Work out the finished part from the listing and answer in its coordinate system (mm). Coordinates: 2 decimals unless noted, no trailing zeros. Write each loop counter-clockwise with the first axis right and the second up, starting at its lowest first coordinate (ties: lowest second). Pieces come first, ordered by that corner, then holes. Notation, with made-up numbers: (-16.75, 12) - (35.25, 12) arc R14 cw to (35.25, 16) - close; hole circle Ø5 at (62, 82). An arc over 180 degrees is marked (long way). Use a Markdown table: item, result. Add a question column.
(1) For a pull along Y with two mould halves and no side action, classify faces 1 (the face through (100.15, 47.07, 2.03)), 2 (the face through (66, 0, 2)) as released by +Y, released by -Y, zero draft, split by the parting line, or undercut.
(2) The part is cut by section B-B, the plane y = 35. Give the vertices of the cut face in (x, z).
(3) The part is cut by section D-D, the plane x = 101.75. Give the vertices of the cut face in (y, z), then the cut area to 3 significant figures.
(4) Find the intervals of material crossed by line 1 (X direction, y = 34, z = 3.25); line 2 (Y direction, x = 53.75, z = 1.45); line 3 (Y direction, x = 101.75, z = 2.45), in increasing order. Write a range as from..to.
(5) The part is cut by section A-A, the plane x = 125. Give the vertices of the cut face in (y, z).
(6) Given pin 1 Ø5 at (x, y) = (89.75, 47) entering from +Z, flat-ended and moving along its own axis, determine where the tip first touches the part or whether it passes through.
(7) The part is cut by section C-C, the plane x = 77.75. Give the vertices of the cut face in (y, z), then the cut area to 3 significant figures.
Autodesk Inventor part; units mm, degrees
ref_plane "YZ Plane" through (0, 0, 0) normal (1, 0, 0) x (0, 1, 0)
ref_plane "XZ Plane" through (0, 0, 0) normal (0, 1, 0) x (-1, 0, 0)
ref_plane "XY Plane" through (0, 0, 0) normal (0, 0, 1) x (1, 0, 0)
sketch "스케치1" plane through (0, 0, 0) normal (0, 0, 1) x (1, 0, 0)
  line L0 (0, 0) -> (0, 58)
  line L1 (0, 58) -> (129.5, 58)
  line L2 (129.5, 58) -> (129.5, 0)
  line L3 (129.5, 0) -> (0, 0)
  dimension "d0" = 58
  dimension "d1" = 129.5
extrude "돌출1" add sketch "스케치1" along normal blind 4
sketch "스케치2" plane through (0, 0, 4) normal (0, 0, 1) x (1, 0, 0)
  line L0 (62.75, 50) -> (62.75, 8)
  line L1 (32.75, 50) -> (57.25, 50)
  line L2 (62.75, 50) -> (69.25, 50)
  line L3 (81.25, 8) -> (81.25, 50)
  line L4 (74.75, 50) -> (81.25, 50)
  line L5 (74.75, 50) -> (74.75, 8)
  line L6 (74.75, 8) -> (81.25, 8)
  circle A0 centre (77.75, 47) radius 1.6
  circle A1 centre (77.75, 11) radius 1.6
  line L7 (93.25, 8) -> (93.25, 50)
  line L8 (86.75, 50) -> (93.25, 50)
  line L9 (86.75, 50) -> (86.75, 8)
  line L10 (86.75, 8) -> (93.25, 8)
  circle A2 centre (89.75, 47) radius 1.6
  circle A3 centre (89.75, 11) radius 1.6
  line L11 (57.25, 8) -> (57.25, 50)
  line L12 (32.75, 50) -> (57.25, 50)
  line L13 (32.75, 50) -> (32.75, 54)
  line L14 (26.75, 54) -> (32.75, 54)
  line L15 (26.75, 4) -> (26.75, 54)
  line L16 (26.75, 4) -> (32.75, 4)
  line L17 (32.75, 4) -> (32.75, 8)
  line L18 (32.75, 8) -> (57.25, 8)
  circle A4 centre (29.75, 47) radius 1.6
  circle A5 centre (29.75, 11) radius 1.6
  circle A6 centre (41.75, 47) radius 1.6
  circle A7 centre (41.75, 11) radius 1.6
  circle A8 centre (53.75, 47) radius 1.6
  circle A9 centre (53.75, 11) radius 1.6
  line L19 (62.75, 8) -> (69.25, 8)
  circle A10 centre (65.75, 47) radius 1.6
  circle A11 centre (65.75, 11) radius 1.6
  circle A12 centre (101.75, 11) radius 1.6
  circle A13 centre (113.75, 11) radius 1.6
  circle A14 centre (113.75, 47) radius 1.6
  circle A15 centre (101.75, 47) radius 1.6
  circle A16 centre (5.75, 11) radius 1.6
  circle A17 centre (5.75, 47) radius 1.6
  line L20 (113.75, 11) -> (113.75, 47)
  line L21 (5.75, 11) -> (5.75, 47)
  line L22 (129.5, 0) -> (129.5, 58)
  line L23 (0, 0) -> (129.5, 0)
  line L24 (0, 58) -> (0, 0)
  line L25 (113.75, 47) -> (132.75, 47)
  line L26 (113.75, 11) -> (132.75, 11)
  line L27 (132.75, 11) -> (132.75, 47)
  line L28 (5.75, 47) -> (-3.25, 47)
  line L29 (-3.25, 47) -> (-3.25, 11)
  line L30 (-3.25, 11) -> (5.75, 11)
  line L31 (-3.25, 29) -> (132.75, 29)
  line L32 (0, 58) -> (-3.25, 58)
  line L33 (-3.25, 58) -> (-3.25, 0)
  line L34 (-3.25, 0) -> (0, 0)
  dimension "d27" = 19
  dimension "d28" = 9
  dimension "d30" = 3.25
  dimension "d31" = 21
  dimension "d32" = 5.5
  dimension "d34" = 3.25
extrude "돌출2" cut sketch "스케치2" against normal blind 6 contours L21 L30 A16 | A16 L30 L21 | L21 L28 A17 | A17 L28 L21 | L20 L26 A13 | A13 L26 L20 | L20 L25 A14 | A14 L25 L20 | A0 | A1 | A2 | A3 | A4 | A5 | A6 | A7 | A8 | A9 | A10 | A11 | A12 | A15
sketch "스케치3" plane through (0, 0, 4) normal (0, 0, 1) x (1, 0, 0)
  circle A0 centre (29.75, 47) radius 1.6
  circle A1 centre (41.75, 11) radius 1.6
  circle A2 centre (89.75, 11) radius 1.6
  circle A3 centre (101.75, 47) radius 1.6
  circle A4 centre (113.75, 11) radius 1.6
  circle A5 centre (89.75, 47) radius 1.6
  circle A6 centre (77.75, 11) radius 1.6
  circle A7 centre (29.75, 11) radius 1.6
  circle A8 centre (5.75, 47) radius 1.6
  circle A9 centre (41.75, 47) radius 1.6
  circle A10 centre (53.75, 11) radius 1.6
  circle A11 centre (65.75, 47) radius 1.6
  circle A12 centre (113.75, 47) radius 1.6
  circle A13 centre (101.75, 11) radius 1.6
  circle A14 centre (77.75, 47) radius 1.6
  circle A15 centre (65.75, 11) radius 1.6
  circle A16 centre (53.75, 47) radius 1.6
  circle A17 centre (5.75, 11) radius 1.6
  line L0 (129.5, 58) -> (0, 58)
  line L1 (0, 58) -> (0, 0)
  line L2 (0, 0) -> (129.5, 0)
  line L3 (129.5, 0) -> (129.5, 58)
extrude "돌출3" add sketch "스케치3" against normal blind 4 contours A4 | A8 | A12 | A17
sketch "스케치4" plane through (0, 0, 4) normal (0, 0, 1) x (1, 0, 0)
  line L0 (129.5, 58) -> (0, 58)
  line L1 (4.5, 58) -> (4.5, 0) construction
  line L2 (0, 0) -> (129.5, 0)
  line L3 (0, 58) -> (0, 0)
  line L4 (64.75, 58) -> (64.75, 0) construction
  circle A0 centre (4.5, 51) radius 1.6
  circle A1 centre (4.5, 40) radius 1.6
  circle A2 centre (4.5, 18) radius 1.6
  circle A3 centre (4.5, 7) radius 1.6
  circle A4 centre (125, 51) radius 1.6
  circle A5 centre (125, 40) radius 1.6
  circle A6 centre (125, 18) radius 1.6
  circle A7 centre (125, 7) radius 1.6
  dimension "d10" = 4.5
  dimension "d11" = 3.2
  dimension "d12" = 3.2
  dimension "d13" = 3.2
  dimension "d14" = 3.2
  dimension "d15" = 11
  dimension "d16" = 22
  dimension "d17" = 11
  dimension "d18" = 7
extrude "돌출4" cut sketch "스케치4" against normal blind 4
sketch "스케치5" plane through (0, 0, 4) normal (0, 0, 1) x (1, 0, 0)
  line L0 (116.0982, 37) -> (116.0982, 21)
  line L1 (16.0982, 21) -> (16.0982, 37)
  line L2 (0, 0) -> (129.5, 0)
  arc A0 (18.0982, 39) -> (16.0982, 37) centre (18.0982, 37) ccw
  arc A1 (16.0982, 21) -> (18.0982, 19) centre (18.0982, 21) ccw
  arc A2 (116.0982, 37) -> (114.0982, 39) centre (114.0982, 37) ccw
  arc A3 (114.0982, 19) -> (116.0982, 21) centre (114.0982, 21) ccw
  line L3 (66.0982, 39) -> (66.0982, 19)
  line L4 (46.0982, 37) -> (46.0982, 21)
  line L5 (86.0982, 37) -> (86.0982, 21)
  line L6 (18.0982, 39) -> (44.0982, 39)
  line L7 (88.0982, 39) -> (114.0982, 39)
  line L8 (114.0982, 19) -> (88.0982, 19)
  line L9 (44.0982, 19) -> (18.0982, 19)
  arc A4 (46.0982, 37) -> (44.0982, 39) centre (44.0982, 37) ccw
  arc A5 (44.0982, 19) -> (46.0982, 21) centre (44.0982, 21) ccw
  arc A6 (86.0982, 21) -> (88.0982, 19) centre (88.0982, 21) ccw
  arc A7 (88.0982, 39) -> (86.0982, 37) centre (88.0982, 37) ccw
  point P0 (16.0982, 39)
  point P1 (116.0982, 19)
  point P2 (116.0982, 39)
  dimension "d35" = 100
  dimension "d36" = 20
  dimension "d38" = 2
  dimension "d41" = 20
  dimension "d42" = 20
  dimension "d43" = 2
extrude "돌출5" cut sketch "스케치5" against normal blind 4
sketch "스케치6" plane through (0, 0, 4) normal (0, 0, 1) x (1, 0, 0)
  line L0 (81.0982, 41.5) -> (81.0982, 16.5) construction
  line L1 (81.0982, 16.5) -> (51.0982, 16.5) construction
  line L2 (51.0982, 16.5) -> (51.0982, 41.5) construction
  line L3 (51.0982, 41.5) -> (81.0982, 41.5) construction
  circle A0 centre (81.0982, 41.5) radius 1.25
  circle A1 centre (81.0982, 16.5) radius 1.25
  circle A2 centre (51.0982, 41.5) radius 1.25
  circle A3 centre (51.0982, 16.5) radius 1.25
  line L4 (46.0982, 37) -> (46.0982, 21)
  line L5 (129.5, 58) -> (0, 58)
  point P0 (0, 0)
  point P1 (66.0982, 29)
  dimension "d44" = 25
  dimension "d45" = 30
  dimension "d46" = 15
  dimension "d47" = 12.5
  dimension "d48" = 2.5
  dimension "d49" = 2.5
  dimension "d50" = 2.5
  dimension "d51" = 2.5
  dimension "d52" = 5
  dimension "d53" = 16.5
extrude "돌출6" cut sketch "스케치6" against normal blind 10
chamfer "모따기1" distance 1.6 angle 45 10 edges at (52.15, 47, 4) (40.15, 47, 4) (64.15, 47, 4) (76.15, 47, 4) (88.15, 47, 4) (88.15, 11, 4) (76.15, 11, 4) (64.15, 11, 4) (52.15, 11, 4) (40.15, 11, 4)
properties part number "조인트3받침_6T" material "알루미늄 6061"
Model answer:
| question | item | result |
|---|---|---|
| 1 | face 1 | undercut |
| 1 | face 2 | released by -Y |
| 2 | outline | (0, 0) - (16.1, 0) - (16.1, 4) - (0, 4) - close; (46.1, 0) - (86.1, 0) - (86.1, 4) - (46.1, 4) - close; (116.1, 0) - (129.5, 0) - (129.5, 4) - (116.1, 4) - close |
| 3 | outline | (0, 0) - (9.4, 0) - (9.4, 4) - (0, 4) - close; (12.6, 0) - (19, 0) - (19, 4) - (12.6, 4) - close; (39, 0) - (45.4, 0) - (45.4, 4) - (39, 4) - close; (48.6, 0) - (58, 0) - (58, 4) - (48.6, 4) - close |
| 3 | area | 126 mm^2 |
| 4 | line 1 | 0..16.1, 46.1..86.1, 116.1..129.5 |
| 4 | line 2 | 0..9.4, 12.6..45.4, 48.6..58 |
| 4 | line 3 | 0..9.4, 12.6..19, 39..45.4, 48.6..58 |
| 5 | outline | (0, 0) - (5.4, 0) - (5.4, 4) - (0, 4) - close; (8.6, 0) - (16.4, 0) - (16.4, 4) - (8.6, 4) - close; (19.6, 0) - (38.4, 0) - (38.4, 4) - (19.6, 4) - close; (41.6, 0) - (49.4, 0) - (49.4, 4) - (41.6, 4) - close; (52.6, 0) - (58, 0) - (58, 4) - (52.6, 4) - close |
| 6 | pin 1 | z = 3.3 |
| 7 | outline | (0, 0) - (9.4, 0) - (9.4, 2.4) - (7.8, 4) - (0, 4) - close; (12.6, 0) - (45.4, 0) - (45.4, 2.4) - (43.8, 4) - (14.2, 4) - (12.6, 2.4) - close; (48.6, 0) - (58, 0) - (58, 4) - (50.2, 4) - (48.6, 2.4) - close |
| 7 | area | 201 mm^2 |
